Source: CAD feature listing. Evaluate the final solid. Frame: model axes, mm. Face numbers are marked on the shaded views. A direction names the side the tool comes from. Give positions to 0.01 mm unless a question says otherwise; leave off trailing zeros. Order: outer loops, then holes, each group sorted by start corner. A loop starts at its lowest first (then second) coordinate and runs counter-clockwise, first axis right, second up. Notation, with made-up numbers: (-12, 20.25) - (27, 20.25) arc R24 cw to (27, 43.25) - close; hole circle Ø2 at (58, 48.5). An arc over 180 degrees is marked (long way). One line per item, written item: value. Start each with the question number.
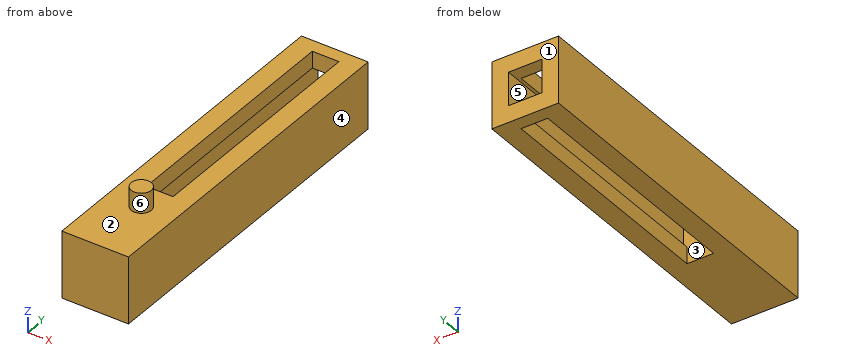
from build123d import *

# Parameters (mm, degrees)
F0_W     = 63.5
F0_H     = 330.2
F0_W_2   = 25.4
F0_H_2   = 228.6
F1_DEPTH = 31.75
F2_W     = 31.75
F2_H     = 31.75
F3_DEPTH = 241.3
F4_R     = 9.525
F5_DEPTH = 19.05


with BuildPart() as f1:
    # F0 (on Top) → F1 (new body, symmetric)
    with BuildSketch(Plane.XY):
        Rectangle(F0_W, F0_H)
        with Locations((0, 38.1)):
            Rectangle(F0_W_2, F0_H_2, mode=Mode.SUBTRACT)
    extrude(amount=F1_DEPTH, both=True)

    # F2 (on face) → F3 (cut)
    with BuildSketch(Plane(origin=(0, 165.1, 0), x_dir=(-1, 0, 0), z_dir=(0, 1, 0))):
        Rectangle(F2_W, F2_H)
    extrude(amount=-F3_DEPTH, mode=Mode.SUBTRACT)

    # F4 (on face) → F5 (join)
    with BuildSketch(Plane.XY.offset(31.75)):
        with Locations((0, -101.6)):
            Circle(F4_R)
    extrude(amount=F5_DEPTH)


solid = f1.part
1. Section C-C on y = -101.6. Return the cut outline in (x, z) (3 decimals).
2. Contact query for flat-ended pins moving along their axis: pin 1 Ø16 at (x, y) = (1, 85.5) entering from +Z; pin 2 Ø6 at (x, y) = (-25, -4) entering from +Z. Output: stop coordinate, or through.
3. Set-up query: the marked faces 4, 5 and 6. Return all of +Z, -Z, +X, -X, +Y, -Y with unobstructed straight access to the full face (end or side cutting, diameter ignored); none if empty.
4. Section B-B on x = 0. Return the cut outline in (y, z) (3 decimals).
5. Section A-A on y = -64. Return the cut outline in (x, z) (3 decimals).
6. Ray query, L1, parallel to X at y = 81.5, z = -16.5; L2, parallel to X at y = 109.5, z = -7.5 (3 decimals); L3, parallel to Y at x = 8, z = 15. Return the intervals inside material, ascending.
7. Draft query along Y for the marked faces 1, 2 and 3. Return one class per face: pulls with the +Y half, pulls with the -Y half, needs draft (parallel to the pull), parting line crosses it, or undercut.
8. Section D-D on z = 41. Return the cut outline in (x, y) (3 decimals), then the cut area to 3 significant figures.
Data:
1. outline: (-31.75, -31.75) - (31.75, -31.75) - (31.75, 31.75) - (9.525, 31.75) - (9.525, 50.8) - (-9.525, 50.8) - (-9.525, 31.75) - (-31.75, 31.75) - close
2. pin 1: passes through
2. pin 2: stops at z = 31.75
3. face 4: +Z, -Z, +X, +Y, -Y
3. face 5: +Y
3. face 6: +Z
4. outline: (-165.1, -31.75) - (-76.2, -31.75) - (-76.2, 31.75) - (-92.075, 31.75) - (-92.075, 50.8) - (-111.125, 50.8) - (-111.125, 31.75) - (-165.1, 31.75) - close; (152.4, -31.75) - (165.1, -31.75) - (165.1, -15.875) - (152.4, -15.875) - close; (152.4, 15.875) - (165.1, 15.875) - (165.1, 31.75) - (152.4, 31.75) - close
5. outline: (-31.75, -31.75) - (-12.7, -31.75) - (-12.7, -15.875) - (-15.875, -15.875) - (-15.875, 15.875) - (-12.7, 15.875) - (-12.7, 31.75) - (-31.75, 31.75) - close; (12.7, -31.75) - (31.75, -31.75) - (31.75, 31.75) - (12.7, 31.75) - (12.7, 15.875) - (15.875, 15.875) - (15.875, -15.875) - (12.7, -15.875) - close
6. L1: x = -31.75 to -12.7, 12.7 to 31.75
6. L2: x = -31.75 to -15.875, 15.875 to 31.75
6. L3: y = -165.1 to -76.2
7. face 1: pulls with the +Y half
7. face 2: needs draft
7. face 3: undercut
8. outline: circle Ø19.05 at (0, -101.6)
8. area: 285 mm2
